Autodesk Fusion 360 part; units mm, degrees
sketch "Sketch1" plane through (0, 0, 0) normal (0, 0, 1) x (1, 0, 0)
  line L0 (0, 0) -> (38.8, 0)
  line L1 (38.8, 0) -> (38.8, 10)
  line L2 (38.8, 10) -> (36.15, 10)
  line L3 (36.15, 10) -> (36.15, 15.3)
  line L4 (36.15, 15.3) -> (38.8, 15.3)
  line L5 (38.8, 15.3) -> (38.8, 27.3)
  line L6 (38.8, 27.3) -> (36.15, 27.3)
  line L7 (36.15, 27.3) -> (36.15, 32.6)
  line L8 (36.15, 32.6) -> (38.8, 32.6)
  line L9 (38.8, 32.6) -> (38.8, 42.6)
  line L10 (38.8, 42.6) -> (64.2, 42.6)
  line L11 (64.2, 42.6) -> (64.2, 55.3)
  line L12 (64.2, 55.3) -> (0, 55.3)
  line L13 (0, 55.3) -> (0, 0)
  dimension "d1" = 38.8
  dimension "d2" = 10
  dimension "d3" = 2.65
  dimension "d4" = 5.3
  dimension "d5" = 2.65
  dimension "d7" = 12
  dimension "d8" = 2.65
  dimension "d9" = 5.3
  dimension "d10" = 2.65
  dimension "d11" = 10
  dimension "d12" = 25.4
  dimension "d13" = 12.7
revolve "Revolve1" add sketch "Sketch1" angle 360 about axis through (0, 55.3, 0) along (0, -1, 0)
sketch "Sketch2" plane through (0, 55.3, 0) normal (0, 1, 0) x (-1, 0, 0)
  circle A0 centre (0, 0) radius 64.2
sketch "Sketch3" plane through (0, 55.3, 0) normal (0, 1, 0) x (-1, 0, 0)
  line L0 (-51.05, 0) -> (-54.25, 0)
  circle A0 centre (-54.25, 0) radius 3.2
  line L1 (51.05, 0) -> (54.25, 0)
  circle A1 centre (54.25, 0) radius 3.2
  dimension "d15" = 54.25
  dimension "d16" = 6.4
  dimension "d17" = 54.25
  dimension "d18" = 6.4
hole "Hole1" at (54.25, 55.3, 0) direction (0, -1, 0) diameter 6.4 depth 100 tip angle 118
sketch "Sketch4" plane through (0, 55.3, 0) normal (0, 1, 0) x (-1, 0, 0)
  line L0 (51.05, 0) -> (54.25, 0)
  circle A0 centre (54.25, 0) radius 3.2
  dimension "d22" = 54.25
  dimension "d23" = 6.4
hole "Hole2" at (-54.25, 55.3, 0) direction (0, -1, 0) diameter 6.4 depth 100 tip angle 118
Part model, mm, in its own coordinate system. A direction names the side the tool comes from. Give positions to 0.01 mm unless a question says otherwise; leave off trailing zeros. Write each loop counter-clockwise with the first axis right and the second up, starting at its lowest first coordinate (ties: lowest second). Pieces come first, ordered by that corner, then holes. Notation, with made-up numbers: (-39.5, 81.5) -> (-7.5, 81.5) arc R19 cw to (-7.5, 102.5) -> close; hole circle Ø9 at (82, 25). An arc over 180 degrees is marked (long way). Put each result on its own line as item: value. Start each with the question number.
Item 1: Which spindle directions (+Z, -Z, +X, -X, +Y, -Y) get a long thin tool onto all of the face, cutting with end or side? Do faces 5 (the face through (37.01, 5.07, -11.65)), 6 (the face through (26, 32.6, -26)), 7 (the face through (51.077, 48.861, -0.417)). Say none if no direction does.
Item 2: Cut at B-B (x = -54.25). List the corners of the cut face in (y, z).
Item 3: Cut at C-C (x = 0). List the corners of the cut face in (y, z), then the cut area to 3 significant figures.
Item 4: Cut at D-D (z = -28). List the corners of the cut face in (x, y).
Item 5: Pin check, flat tips, straight feed: pin 1 Ø5 at (x, y) = (-31.5, 22.5) entering from +Z; pin 2 Ø8 at (x, y) = (10, 31.5) entering from -Z; pin 3 Ø10 at (x, y) = (-12, 46.5) entering from -Z. Stop position of each tip, or through.
Item 6: Cut at A-A (z = 0). State how many separate pieces and enclosed holes the cut face has, then the cut area to 3 significant figures.
Item 7: Pull direction Y, two halves, no side cores. Call faces 1 (the face through (28, 42.6, -28)), 2 (the face through (-1, 55.3, 1)), 3 (the face through (26, 27.3, -26)), 4 (the face through (-57.423, 48.861, -0.417)): pulls with the +Y half, pulls with the -Y half, needs draft (parallel to the pull), parting line crosses it, or undercut.
Item 8: Wall check: L1, parallel to Y at x = -38, z = -6; L2, parallel to Y at x = 33, z = -29; L3, parallel to Z at x = -56, y = 44.5. Give the ranges that are in metal, low to high. Write a range as [from, to].
Answer list:
1. face 5: -Y
1. face 6: none
1. face 7: +Y, -Y
2. outline: (42.6, -34.33) -> (55.3, -34.33) -> (55.3, -3.2) -> (42.6, -3.2) -> close; (42.6, 3.2) -> (55.3, 3.2) -> (55.3, 34.33) -> (42.6, 34.33) -> close
3. outline: (0, -38.8) -> (10, -38.8) -> (10, -36.15) -> (15.3, -36.15) -> (15.3, -38.8) -> (27.3, -38.8) -> (27.3, -36.15) -> (32.6, -36.15) -> (32.6, -38.8) -> (42.6, -38.8) -> (42.6, -64.2) -> (55.3, -64.2) -> (55.3, 64.2) -> (42.6, 64.2) -> (42.6, 38.8) -> (32.6, 38.8) -> (32.6, 36.15) -> (27.3, 36.15) -> (27.3, 38.8) -> (15.3, 38.8) -> (15.3, 36.15) -> (10, 36.15) -> (10, 38.8) -> (0, 38.8) -> close
3. area: 4,880 mm2
4. outline: (-57.77, 42.6) -> (-26.86, 42.6) -> (-26.86, 32.6) -> (-22.87, 32.6) -> (-22.87, 27.3) -> (-26.86, 27.3) -> (-26.86, 15.3) -> (-22.87, 15.3) -> (-22.87, 10) -> (-26.86, 10) -> (-26.86, 0) -> (26.86, 0) -> (26.86, 10) -> (22.87, 10) -> (22.87, 15.3) -> (26.86, 15.3) -> (26.86, 27.3) -> (22.87, 27.3) -> (22.87, 32.6) -> (26.86, 32.6) -> (26.86, 42.6) -> (57.77, 42.6) -> (57.77, 55.3) -> (-57.77, 55.3) -> close
5. pin 1: stops at z = 25.78
5. pin 2: stops at z = -38.31
5. pin 3: stops at z = -63.82
6. separate pieces: 3
6. enclosed holes: 0
6. area: 4,720 mm2
7. face 1: pulls with the -Y half
7. face 2: pulls with the +Y half
7. face 3: undercut
7. face 4: needs draft
8. L1: y = [0, 10], [15.3, 27.3], [32.6, 55.3]
8. L2: y = [42.6, 55.3]
8. L3: z = [-31.39, -2.68], [2.68, 31.39]
